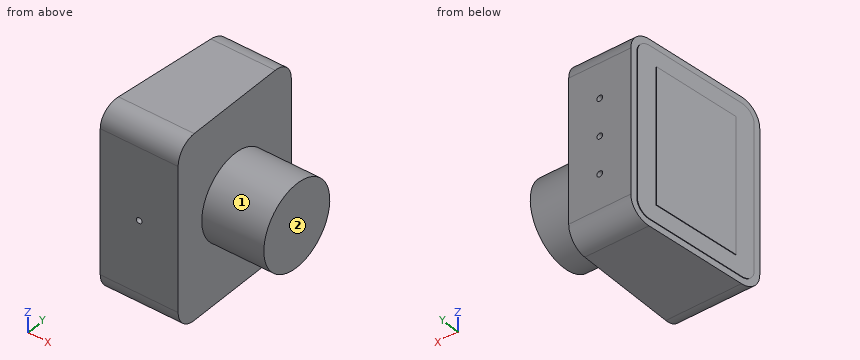
```python
from build123d import *

# Parameters (mm, degrees)
EXTRUDE_1_DEPTH           = 165
FILLET_1_R                = 18
SKETCH_2_R                = 37
EXTRUDE_2_DEPTH           = 55
HOLE_WIZARD_1_4_201_D     = 5.1054
HOLE_WIZARD_1_4_201_DEPTH = 12
HOLE_WIZARD_1_4_201_TIP   = 1.533816902
HOLE_WIZARD_1_4_202_D     = 5.1054
HOLE_WIZARD_1_4_202_DEPTH = 12
HOLE_WIZARD_1_4_202_TIP   = 1.533816902
EXTRUDE_3_DEPTH           = 1
SKETCH_10_OUTSIDE_W       = 215.504
SKETCH_10_OUTSIDE_H       = 190.363
SKETCH_10_OUTSIDE_W_2     = 121.90164915
SKETCH_10_OUTSIDE_H_2     = 79.127933184
CUT_EXTRUDE_1_DEPTH       = 0.5


with BuildPart() as part:
    # Эскиз1 → Бобышка-Вытянуть1 (new body)
    with BuildSketch(Plane.XY):
        Polygon((0, 0), (0, 127), (-55, 127), (-69, 0), align=None)
    extrude(amount=EXTRUDE_1_DEPTH)

    # Скругление1
    fillet_1_edges = [part.edges().sort_by_distance(p)[0] for p in [
        (-27.5, 127, 165),
        (-34.5, 0, 165),
        (-27.5, 127, 0),
        (-34.5, 0, 0),
    ]]
    fillet(fillet_1_edges, radius=FILLET_1_R)

    # Эскиз2 → Бобышка-Вытянуть2 (add)
    with BuildSketch(Plane(origin=(0, 0, 0), x_dir=(0, 0, -1), z_dir=(1, 0, 0))):
        with Locations((-82.5, 63.5)):
            Circle(SKETCH_2_R)
    extrude(amount=EXTRUDE_2_DEPTH)

    # Отверстие обработанное метчиком 1/4-201
    with Locations(Plane(origin=(0, 127, 0), x_dir=(1, 0, 0), z_dir=(0, 1, 0))):
        with Locations((-27.5, -49.1), (-27.5, -82.5), (-27.5, -115.9)):
            Hole(HOLE_WIZARD_1_4_201_D / 2, depth=HOLE_WIZARD_1_4_201_DEPTH)
            with Locations((0, 0, -(HOLE_WIZARD_1_4_201_DEPTH + HOLE_WIZARD_1_4_201_TIP / 2))):  # 118° drill point
                Cone(0, HOLE_WIZARD_1_4_201_D / 2, HOLE_WIZARD_1_4_201_TIP, mode=Mode.SUBTRACT)

    # Отверстие обработанное метчиком 1/4-202
    with Locations(Plane(origin=(0, 0, 0), x_dir=(-1, 0, 0), z_dir=(0, -1, 0))):
        with Locations((34.5, -82.5)):
            Hole(HOLE_WIZARD_1_4_202_D / 2, depth=HOLE_WIZARD_1_4_202_DEPTH)
            with Locations((0, 0, -(HOLE_WIZARD_1_4_202_DEPTH + HOLE_WIZARD_1_4_202_TIP / 2))):  # 118° drill point
                Cone(0, HOLE_WIZARD_1_4_202_D / 2, HOLE_WIZARD_1_4_202_TIP, mode=Mode.SUBTRACT)

    # Эскиз9 → Бобышка-Вытянуть3 (add)
    with BuildSketch(Plane(origin=(-68.171577335, 7.514977029, 0), x_dir=(0, 0, 1), z_dir=(-0.99397881, 0.109572467, 0))):
        with BuildLine():
            Line((18, -1.560500239), (147, -1.560500239))
            add(Edge.make_bspline(
                [(147, -1.560500239), (147.795969048, -1.560500239), (148.578437938, -1.48137479), (149.732739087, -1.248968925), (150.114248167, -1.152405098), (150.870602957, -0.920222923), (151.246130664, -0.784060546), (152.337830508, -0.325667383), (153.027835256, 0.048140187), (154.006731596, 0.710119453), (154.325036907, 0.948994101), (154.935136946, 1.45617868), (155.225430555, 1.722967352), (156.053427969, 2.561683199), (156.548653408, 3.171597982), (157.20432669, 4.164420075), (157.407043585, 4.507004661), (157.774884438, 5.203781035), (158.107288123, 5.915340648), (158.369821072, 6.656048071), (158.596915662, 7.41153923), (158.6930429, 7.79849924), (158.923007799, 8.965817399), (159, 9.752769129), (159, 10.548537722)],
                knots=[0, 0, 0, 0, 0.125, 0.125, 0.1875, 0.1875, 0.25, 0.25, 0.375, 0.375, 0.4375, 0.4375, 0.5, 0.5, 0.625, 0.625, 0.6875, 0.6875, 0.75, 0.8125, 0.8125, 0.875, 0.875, 1, 1, 1, 1], degree=3))
            Line((159, 10.548537722), (159, 102.099785192))
            add(Edge.make_bspline(
                [(159, 102.099785192), (159, 102.89567677), (158.92299313, 103.678477169), (158.69658927, 104.833825846), (158.602503189, 105.215776987), (158.376242963, 105.973204292), (158.243333402, 106.350026622), (157.795055135, 107.447066101), (157.429092547, 108.141223603), (156.564023929, 109.455731539), (156.059486079, 110.079699577), (154.955465788, 111.199609881), (154.352820703, 111.702413635), (153.371115524, 112.368877293), (153.029785995, 112.576618568), (152.335786173, 112.953165195), (151.627066488, 113.293348749), (150.889392409, 113.562005098), (150.137062243, 113.794455923), (149.752332485, 113.89282261), (148.583675335, 114.129662505), (147.796097323, 114.208823153), (147, 114.208823153)],
                knots=[0, 0, 0, 0, 0.125, 0.125, 0.1875, 0.1875, 0.25, 0.25, 0.375, 0.375, 0.5, 0.5, 0.625, 0.625, 0.6875, 0.6875, 0.75, 0.8125, 0.8125, 0.875, 0.875, 1, 1, 1, 1], degree=3))
            Line((147, 114.208823153), (18, 114.208823153))
            add(Edge.make_bspline(
                [(18, 114.208823153), (17.204030952, 114.208823153), (16.421562062, 114.129697705), (15.267260913, 113.897291839), (14.885751833, 113.800728013), (14.129397043, 113.568545837), (13.753869336, 113.43238346), (12.662169492, 112.973990297), (11.972164744, 112.600182727), (10.993268404, 111.938203462), (10.674963093, 111.699328814), (10.064863054, 111.192144234), (9.774569445, 110.925355563), (8.946572031, 110.086639716), (8.451346592, 109.476724932), (7.79567331, 108.48390284), (7.592956415, 108.141318253), (7.225115562, 107.444541879), (6.892711877, 106.732982266), (6.630178928, 105.992274843), (6.403084338, 105.236783685), (6.3069571, 104.849823675), (6.076992201, 103.682505516), (6, 102.895553785), (6, 102.099785192)],
                knots=[0, 0, 0, 0, 0.125, 0.125, 0.1875, 0.1875, 0.25, 0.25, 0.375, 0.375, 0.4375, 0.4375, 0.5, 0.5, 0.625, 0.625, 0.6875, 0.6875, 0.75, 0.8125, 0.8125, 0.875, 0.875, 1, 1, 1, 1], degree=3))
            Line((6, 102.099785192), (6, 10.548537722))
            add(Edge.make_bspline(
                [(6, 10.548537722), (6, 9.752646144), (6.07700687, 8.969845746), (6.30341073, 7.814497069), (6.397496811, 7.432545928), (6.623757037, 6.675118622), (6.756666598, 6.298296292), (7.204944865, 5.201256813), (7.570907453, 4.507099312), (8.435976071, 3.192591376), (8.940513921, 2.568623338), (10.044534212, 1.448713034), (10.647179297, 0.945909279), (11.628884476, 0.279445622), (11.970214005, 0.071704346), (12.664213827, -0.30484228), (13.372933512, -0.645025835), (14.110607591, -0.913682184), (14.862937757, -1.146133008), (15.247667515, -1.244499696), (16.416324665, -1.48133959), (17.203902677, -1.560500239), (18, -1.560500239)],
                knots=[0, 0, 0, 0, 0.125, 0.125, 0.1875, 0.1875, 0.25, 0.25, 0.375, 0.375, 0.5, 0.5, 0.625, 0.625, 0.6875, 0.6875, 0.75, 0.8125, 0.8125, 0.875, 0.875, 1, 1, 1, 1], degree=3))
        make_face()
    extrude(amount=EXTRUDE_3_DEPTH)

    # Эскиз10 outside → Вырез-Вытянуть1 (cut)
    with BuildSketch(Plane(origin=(-69.165556145, 7.624549496, 0), x_dir=(0, 0, 1), z_dir=(-0.99397881, 0.109572467, 0))):
        with Locations((82.5, 62.3325)):
            Rectangle(SKETCH_10_OUTSIDE_W, SKETCH_10_OUTSIDE_H)
        with Locations((82.5, 56.324161457)):
            Rectangle(SKETCH_10_OUTSIDE_W_2, SKETCH_10_OUTSIDE_H_2, mode=Mode.SUBTRACT)
    extrude(amount=-CUT_EXTRUDE_1_DEPTH, mode=Mode.SUBTRACT)


solid = part.part
```
For this review, take the finished solid that the model builds, in its own axes (mm). Face numbers are marked on the shaded views. A direction names the side the tool comes from. Coordinates: 2 decimals unless noted, no trailing zeros. Order: outer loops, then holes, each group sorted by start corner. A loop starts at its lowest first (then second) coordinate and runs counter-clockwise, first axis right, second up. Notation, with made-up numbers: (74, 59) - (116, 59) arc R30 ccw to (116, 95) - close; hole circle Ø5 at (15, 66). An arc over 180 degrees is marked (long way). Answer as a JSON object with one key per item and string values. Group by question number.
1. We need section A-A on y = 31.5. State the section outline as (x, z) points, then the cut area to 3 significant figures.
2. We need section C-C on x = 31. State the section outline as (y, z) points, then the cut area to 3 significant figures.
3. For probe 1 along Z at (x, y) = (-27, 123); probe 2 along Z at (x, y) = (-27.5, 121.5); probe 3 along Z at (x, y) = (-34.5, 8.75), list the stretches that pass through material, from the lowest coordinate up.
4. Clearance check with flat-ended pins moving along their axes: P1, Ø12, axis at x = 42.5, z = 67, coming from the -Y side; P2, Ø12, axis at x = -52.5, y = 114, coming from the -Z side; P3, Ø3, axis at x = -64, y = 62.5, coming from the +Z side; P4, Ø5.5, axis at x = -64.5, y = 74, coming from the +Z side. State where each tip first meets the part, or that it passes through.
5. We need section B-B on z = 110.5. State the section outline as (x, y) points, then the cut area to 3 significant figures.
6. For the marked faces 1 and 2, list the 3-axis set-ups (+Z, -Z, +X, -X, +Y, -Y) from which the entire face can be reached by the end or side of a thin tool; tool diameter is ignored.
Final values:
{
 "1": {"outline": "(-66.53, 21.55) - (-66.03, 21.55) - (-66.03, 6) - (-65.53, 6) - (-65.53, 0) - (0, 0) - (0, 63.93) - (55, 63.93) - (55, 101.07) - (0, 101.07) - (0, 165) - (-65.53, 165) - (-65.53, 159) - (-66.03, 159) - (-66.03, 143.45) - (-66.53, 143.45) - close", "area": "13,000 mm²"},
 "2": {"outline": "circle Ø74 at (63.5, 82.5)", "area": "4,300 mm²"},
 "3": {"probe 1": "6.69 to 46.6, 51.6 to 80, 85 to 113.4, 118.4 to 158.31", "probe 2": "5.05 to 46.55, 51.65 to 79.95, 85.05 to 113.35, 118.45 to 159.95", "probe 3": "2.56 to 79.95, 85.05 to 162.44"},
 "4": {"P1": "y = 27.74", "P2": "z = 0", "P3": "z = 159", "P4": "z = 143.45"},
 "5": {"outline": "(-69, 0) - (0, 0) - (0, 39.31) - (55, 39.31) - (55, 87.69) - (0, 87.69) - (0, 127) - (-55, 127) - (-55.66, 121.04) - (-56.15, 121.09) - (-58.16, 102.88) - (-58.66, 102.94) - (-67.33, 24.28) - (-66.83, 24.23) - (-68.84, 6.02) - (-68.34, 5.96) - close", "area": "10,600 mm²"},
 "6": {"face 1": "+X", "face 2": "+Z, -Z, +X, +Y, -Y"}
}
